from build123d import *

# Parameters (mm, degrees)
F1_DEPTH      = 5
F1_DEPTH_BACK = 5
F2_ANGLE      = 30
F3_DEPTH      = 25
F3_DEPTH_BACK = 25
F5_COUNT      = 6
F6_DEPTH      = 8.3061645655
F6_DEPTH_BACK = 8.3061645655


with BuildPart() as f1:
    # F0 (on Top) → F1 (new body, two sides)
    with BuildSketch(Plane.XY) as f1_sk:
        with BuildLine():
            ThreePointArc((28.9777747887, 7.7645713531), (29.7433458412, 3.9157857666), (30, 0))
            ThreePointArc((30, 0), (29.7433458412, -3.9157857666), (28.9777747887, -7.7645713531))
            Line((28.9777747887, -7.7645713531), (96.5925826289, -25.8819045103))
            ThreePointArc((96.5925826289, -25.8819045103), (99.1444861374, -13.052619222), (100, 0))
            ThreePointArc((100, 0), (99.1444861374, 13.052619222), (96.5925826289, 25.8819045103))
            Line((96.5925826289, 25.8819045103), (28.9777747887, 7.7645713531))
        make_face()
        with BuildLine():
            ThreePointArc((28.9777747887, -7.7645713531), (29.7433458412, -3.9157857666), (30, 0))
            ThreePointArc((30, 0), (29.7433458412, 3.9157857666), (28.9777747887, 7.7645713531))
            Line((28.9777747887, 7.7645713531), (14.4888873943, 3.8822856765))
            ThreePointArc((14.4888873943, 3.8822856765), (14.8716729206, 1.9578928833), (15, 0))
            ThreePointArc((15, 0), (14.8716729206, -1.9578928833), (14.4888873943, -3.8822856765))
            Line((14.4888873943, -3.8822856765), (28.9777747887, -7.7645713531))
        make_face()
    extrude(amount=F1_DEPTH)
    extrude(f1_sk.sketch, amount=-F1_DEPTH_BACK)


with BuildPart() as f1_1:
    # F2: moved
    add(f1.part.rotate(Axis((7.5, 0, 0), (1, 0, 0)), F2_ANGLE))

    # F0 (on Top) → F3 (cut, two sides)
    with BuildSketch(Plane.XY) as f3_sk:
        with BuildLine():
            Line((14.4888873943, 3.8822856765), (28.9777747887, 7.7645713531))
            ThreePointArc((28.9777747887, 7.7645713531), (-30, 0), (28.9777747887, -7.7645713531))
            Line((28.9777747887, -7.7645713531), (14.4888873943, -3.8822856765))
            ThreePointArc((14.4888873943, -3.8822856765), (-15, 0), (14.4888873943, 3.8822856765))
        make_face()
        with BuildLine():
            Line((0, 0), (14.4888873943, 3.8822856765))
            ThreePointArc((14.4888873943, 3.8822856765), (-15, 0), (14.4888873943, -3.8822856765))
            Line((14.4888873943, -3.8822856765), (0, 0))
        make_face()
        with BuildLine():
            Line((0, 0), (14.4888873943, -3.8822856765))
            ThreePointArc((14.4888873943, -3.8822856765), (14.8716729206, -1.9578928833), (15, 0))
            Line((15, 0), (0, 0))
        make_face()
        with BuildLine():
            ThreePointArc((15, 0), (14.8716729206, 1.9578928833), (14.4888873943, 3.8822856765))
            Line((14.4888873943, 3.8822856765), (0, 0))
            Line((0, 0), (15, 0))
        make_face()
        with BuildLine():
            ThreePointArc((28.9777747887, -7.7645713531), (29.7433458412, -3.9157857666), (30, 0))
            ThreePointArc((30, 0), (29.7433458412, 3.9157857666), (28.9777747887, 7.7645713531))
            Line((28.9777747887, 7.7645713531), (14.4888873943, 3.8822856765))
            ThreePointArc((14.4888873943, 3.8822856765), (14.8716729206, 1.9578928833), (15, 0))
            ThreePointArc((15, 0), (14.8716729206, -1.9578928833), (14.4888873943, -3.8822856765))
            Line((14.4888873943, -3.8822856765), (28.9777747887, -7.7645713531))
        make_face()
    extrude(amount=-F3_DEPTH, mode=Mode.SUBTRACT)
    extrude(f3_sk.sketch, amount=F3_DEPTH_BACK, mode=Mode.SUBTRACT)


with BuildPart() as f5_1:
    # F5: instance of F1
    add(f1_1.part.rotate(Axis((0, 0, 22.1990030259), (0, 0, 1)), 1 * 360 / F5_COUNT))


with BuildPart() as f5_2:
    # F5: instance of F1
    add(f1_1.part.rotate(Axis((0, 0, 22.1990030259), (0, 0, 1)), 2 * 360 / F5_COUNT))


with BuildPart() as f5_3:
    # F5: instance of F1
    add(f1_1.part.rotate(Axis((0, 0, 22.1990030259), (0, 0, 1)), 3 * 360 / F5_COUNT))


with BuildPart() as f5_4:
    # F5: instance of F1
    add(f1_1.part.rotate(Axis((0, 0, 22.1990030259), (0, 0, 1)), 4 * 360 / F5_COUNT))


with BuildPart() as f5_5:
    # F5: instance of F1
    add(f1_1.part.rotate(Axis((0, 0, 22.1990030259), (0, 0, 1)), 5 * 360 / F5_COUNT))


with BuildPart() as f1_2:
    add(f1_1.part)

    add(f5_1.part)  # F6 merges F5_1

    add(f5_2.part)  # F6 merges F5_2

    add(f5_3.part)  # F6 merges F5_3

    add(f5_4.part)  # F6 merges F5_4

    add(f5_5.part)  # F6 merges F5_5
    # F0 (on Top) → F6 (join, two sides)
    with BuildSketch(Plane.XY) as f6_sk:
        with BuildLine():
            Line((14.4888873943, 3.8822856765), (28.9777747887, 7.7645713531))
            ThreePointArc((28.9777747887, 7.7645713531), (-30, 0), (28.9777747887, -7.7645713531))
            Line((28.9777747887, -7.7645713531), (14.4888873943, -3.8822856765))
            ThreePointArc((14.4888873943, -3.8822856765), (-15, 0), (14.4888873943, 3.8822856765))
        make_face()
        with BuildLine():
            ThreePointArc((28.9777747887, -7.7645713531), (29.7433458412, -3.9157857666), (30, 0))
            ThreePointArc((30, 0), (29.7433458412, 3.9157857666), (28.9777747887, 7.7645713531))
            Line((28.9777747887, 7.7645713531), (14.4888873943, 3.8822856765))
            ThreePointArc((14.4888873943, 3.8822856765), (14.8716729206, 1.9578928833), (15, 0))
            ThreePointArc((15, 0), (14.8716729206, -1.9578928833), (14.4888873943, -3.8822856765))
            Line((14.4888873943, -3.8822856765), (28.9777747887, -7.7645713531))
        make_face()
    extrude(amount=F6_DEPTH)
    extrude(f6_sk.sketch, amount=-F6_DEPTH_BACK)


solid = f1_2.part
Verification items for the finished model (mm, model axes). A direction names the side the tool comes from. Round coordinates to 2 decimals unless told otherwise and drop trailing zeros. Loops run counter-clockwise (first coordinate to the right, second up) from the corner with the lowest first, then second, coordinate; pieces in that order, holes last. Notation, with made-up numbers: (38, 28.25) - (87, 28.25) arc R14 cw to (87, 55.25) - close; hole circle Ø1 at (-5.5, 77). An arc over 180 degrees is marked (long way). Write item = value, one per line.
Q1. Sectioned sample at B-B on y = 39. Record the boundary of the cut face in (x, z).
Here are the results:
outline = (-39.78, 2.86) - (-14.42, -9.82) - (-9.33, -0.82) - (-33.12, 11.07) - close; (9.33, 0.82) - (33.12, -11.07) - (39.78, -2.86) - (14.42, 9.82) - close
Q2. Tool access check on faces 1 (the flat face through (71.72, -2.19, 4.51)), 2 (the flat face through (38.3, -60.71, -4.15)), 3 (the flat face through (-37.76, -61.02, 4.51)), 4 (the flat face through (-71.72, -2.81, -4.15)). Record the directions out of +Z, -Z, +X, -X, +Y, -Y that give a thin tool (end or side, any length) a straight path to the whole face; none if there is none.
Here are the results:
face_1 = +Z, +X
face_2 = -Z, +X
face_3 = +Z, -X
face_4 = -Z, -X
Q3. Sectioned sample at C-C on z = -13. State how many separate pieces and enclosed holes the cut face has, plus the area to 3 significant figures.
Here are the results:
separate_pieces = 6
enclosed_holes = 0
area = 1,000 mm^2
Q4. Depth check by flat-ended pin: pin 1 (4 mm diameter, centred on x = 79, z = -13, fed in from -Y); pin 2 (1.5 mm diameter, centred on y = 13, z = 3.5, fed in from +X); pin 3 (10 mm diameter, centred on y = 47, z = 3.5, fed in from -X). Enter the tip coordinate at first touch or a pass-through.
Here are the results:
pin_1 = -18.25
pin_2 = 99.25
pin_3 = -51.68
Q5. Sectioned sample at A-A on x = 0. Record the boundary of the cut face in (y, z), plus the area to 3 significant figures.
Here are the results:
outline = (-30, -8.31) - (-15, -8.31) - (-15, 8.31) - (-30, 8.31) - close; (15, -8.31) - (30, -8.31) - (30, 8.31) - (15, 8.31) - close
area = 498 mm^2
Q6. Material ranges on L1, parallel to Y at x = 0, z = 5.75; L2, parallel to X at y = 0, z = 3; L3, parallel to Y at x = 67, z = 10, recorded low to high.
Here are the results:
L1 = -30 to -15, 15 to 30
L2 = -99.99 to -15, 15 to 99.99
L3 = -73.59 to -69.58, 7.32 to 14.96
